Input: dimensioned drawing with shaded views. Units: mm. Origin: part minimum x, y, z. A direction names the side the tool comes from. Give positions to 0.01 mm unless a question says otherwise; leave off trailing zeros. Write each loop counter-clockwise with the first axis right and the second up, starting at its lowest first coordinate (ties: lowest second). Pieces come first, ordered by that corner, then holes. Notation, with made-up numbers: (-35.5, -16) -> (-27.5, -16) arc R19 ccw to (-27.5, 8) -> close; hole circle Ø2 at (-3.5, 18.5). An arc over 180 degrees is marked (long way). Answer as a JSON object with one key per item and string values. Group by question number.
(1) Section query C-C on x = 20. Output: boundary loops of the cut face in (y, z), plus the area to 3 significant figures.
(2) Section query B-B on z = 24.5. State how many separate pieces and enclosed holes the cut face has, plus the area to 3 significant figures.
(3) Set-up query: the marked faces 1 and 2. Return all of +Z, -Z, +X, -X, +Y, -Y with unobstructed straight access to the full face (end or side cutting, diameter ignored); none if empty.
(4) Contact query for flat-ended pins moving along their axis: pin 1 Ø3 at (x, y) = (44.5, 13) entering from +Z; pin 2 Ø1.2 at (x, z) = (70.5, 21.5) entering from +Y. Output: stop coordinate, or through.
(5) Draft query along Y for the marked faces 3, 4, 5 and 6. Return one class per face: +Y half, -Y half, draft (parallel to the pull), parting line (faces both ways), or undercut.
(6) Material intervals for probe 1 along X at (y, z) = (42.5, 2); probe 2 along Y at (x, z) = (44, 25); probe 3 along X at (y, z) = (53, 22.5), sorted ascending.
(7) Section query A-A on y = 43. Output: boundary loops of the cut face in (x, z).
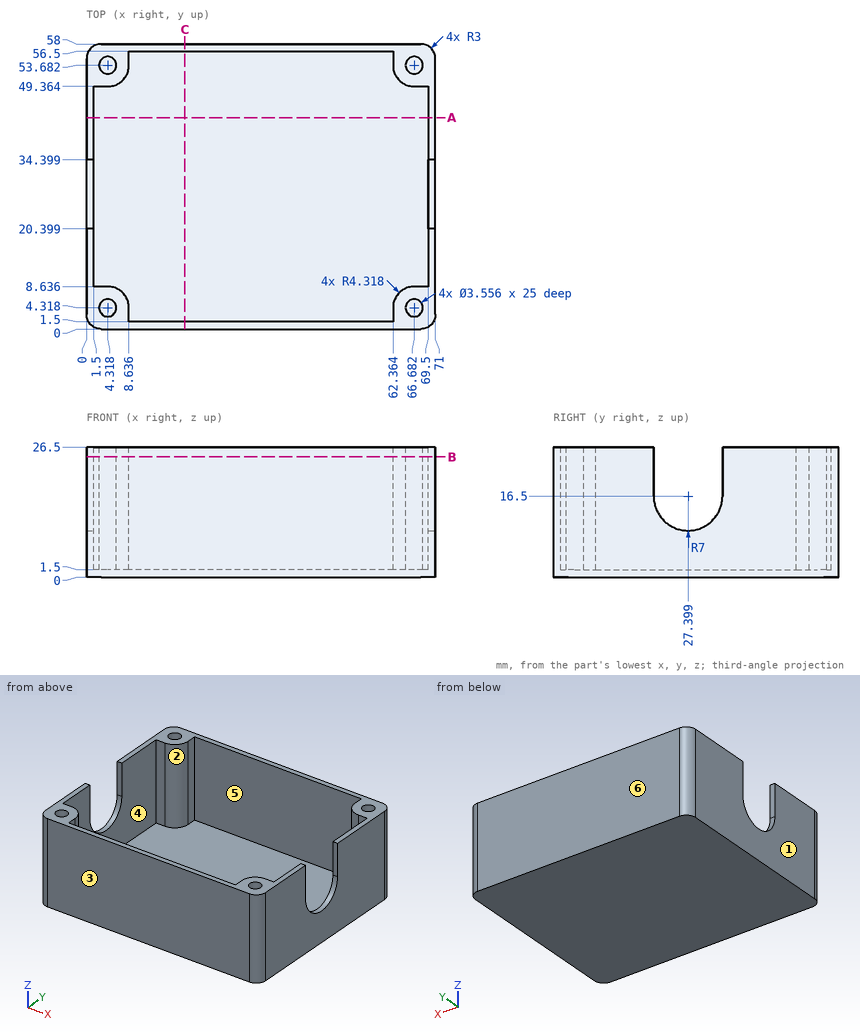
Answer list:
{
 "1": {"outline": "(0, 0) -> (58, 0) -> (58, 26.5) -> (56.5, 26.5) -> (56.5, 1.5) -> (1.5, 1.5) -> (1.5, 26.5) -> (0, 26.5) -> close", "area": "162 mm2"},
 "2": {"separate pieces": "2", "enclosed holes": "4", "area": "476 mm2"},
 "3": {"face 1": "+Z, -Z, -X, +Y, -Y", "face 2": "+Z"},
 "4": {"pin 1": "z = 1.5", "pin 2": "y = 57.32"},
 "5": {"face 3": "-Y half", "face 4": "undercut", "face 5": "undercut", "face 6": "+Y half"},
 "6": {"probe 1": "0 to 1.5, 69.5 to 71", "probe 2": "0 to 1.5, 56.5 to 58", "probe 3": "0 to 2.68, 5.96 to 8.58, 62.42 to 65.04, 68.32 to 71"},
 "7": {"outline": "(0, 0) -> (71, 0) -> (71, 26.5) -> (69.5, 26.5) -> (69.5, 1.5) -> (1.5, 1.5) -> (1.5, 26.5) -> (0, 26.5) -> close"}
}
